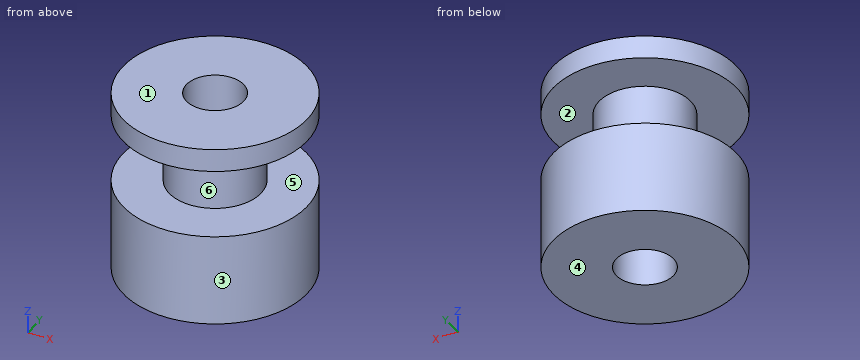
Autodesk Inventor part; units mm, degrees
ref_plane "Work Plane1" through (0, 0, 14) normal (0, 0, 1) x (1, 0, 0)
ref_plane "YZ Plane" through (0, 0, 0) normal (1, 0, 0) x (0, 1, 0)
ref_plane "XZ Plane" through (0, 0, 0) normal (0, 1, 0) x (-1, 0, 0)
sketch "Sketch1" plane through (0, 0, 0) normal (0, 0, 1) x (1, 0, 0)
  circle A0 centre (0, 0) radius 8
  circle A1 centre (0, 0) radius 2.5
  dimension "d0" = 16
  dimension "d3" = 5
extrude "Extrusion1" add sketch "Sketch1" along normal blind 16
ref_plane "Work Plane1" through (0, 0, 14) normal (0, 0, 1) x (1, 0, 0)
sketch "Sketch3" plane through (0, 0, 14) normal (0, 0, 1) x (1, 0, 0)
  circle A0 centre (0, 0) radius 8
  circle A1 centre (0, 0) radius 2.5
  circle A2 centre (0, 0) radius 2.5
  circle A3 centre (0, 0) radius 4
  dimension "d5" = 5
  dimension "d6" = 8
extrude "Extrusion2" cut sketch "Sketch3" against normal blind 6 contours A0
properties part number "pulley-small" material "Aluminum"
Read the model definition and answer for the solid it produces. Units are mm, in the model's axes. Face numbers are marked on the shaded views. A direction names the side the tool comes from. Round coordinates to 2 decimals unless told otherwise and drop trailing zeros. Loops run counter-clockwise (first coordinate to the right, second up) from the corner with the lowest first, then second, coordinate; pieces in that order, holes last.
Q1. Which of the six approach directions +Z, -Z, +X, -X, +Y, -Y give full straight-line access (tool end or side, diameter ignored) to the marked faces 1 and 2?
Q2. Section B-B on y = 5 is taken. Write down the section's boundary in (x, z) (3 decimals).
Q3. Determine the mould class of the marked faces 3, 4, 5 and 6 for opening direction Z: released by +Z, released by -Z, zero draft, split by the parting line, or undercut.
Q4. Consider probe 1 along Y at (x, z) = (0, 10); probe 2 along Z at (x, y) = (5.75, -4); probe 3 along Y at (x, z) = (0, 7.25). Determine where each line is inside the solid, lowest interval first.
Q5. This flat-tipped pin is pushed along its axis until it touches: pin 1 (5 mm diameter, centred on x = -4, z = 3.5, fed in from -Y). Where does it stop, or does it pass through?
Q6. Section A-A on x = -6.75 is taken. Write down the section's boundary in (y, z), and give its area (3 significant figures).
Q7. Section C-C on z = 4.75 is taken. Write down the section's boundary in (x, y), and give its area (3 significant figures).
Q8. Section D-D on x = -2.75 is taken. Write down the section's boundary in (y, z).
Output:
1. face 1: +Z, +X, -X, +Y, -Y
1. face 2: none
2. outline: (-6.245, 0) - (6.245, 0) - (6.245, 8) - (-6.245, 8) - close; (-6.245, 14) - (6.245, 14) - (6.245, 16) - (-6.245, 16) - close
3. face 3: zero draft
3. face 4: released by -Z
3. face 5: undercut
3. face 6: undercut
4. probe 1: y = -4 to -2.5, 2.5 to 4
4. probe 2: z = 0 to 8, 14 to 16
4. probe 3: y = -8 to -2.5, 2.5 to 8
5. pin 1: stops at y = -7.86
6. outline: (-4.29, 0) - (4.29, 0) - (4.29, 8) - (-4.29, 8) - close; (-4.29, 14) - (4.29, 14) - (4.29, 16) - (-4.29, 16) - close
6. area: 85.9 mm2
7. outline: circle Ø16 at (0, 0); hole circle Ø5 at (0, 0)
7. area: 181 mm2
8. outline: (-7.51, 0) - (7.51, 0) - (7.51, 8) - (2.9, 8) - (2.9, 14) - (7.51, 14) - (7.51, 16) - (-7.51, 16) - (-7.51, 14) - (-2.9, 14) - (-2.9, 8) - (-7.51, 8) - close
